Autodesk Inventor part; units mm, degrees
ref_plane "YZ Plane" through (0, 0, 0) normal (1, 0, 0) x (0, 1, 0)
ref_plane "XZ Plane" through (0, 0, 0) normal (0, 1, 0) x (-1, 0, 0)
ref_plane "XY Plane" through (0, 0, 0) normal (0, 0, 1) x (1, 0, 0)
sketch "Sketch1" plane through (0, 0, 0) normal (0, 1, 0) x (-1, 0, 0)
  line L0 (0, 0) -> (-41, 0)
  line L1 (-41, 0) -> (-41, -47)
  line L2 (-41, -47) -> (0, -47)
  line L3 (0, -47) -> (0, 0)
  dimension "d0" = 41
  dimension "d1" = 47
extrude "Extrusion1" add sketch "Sketch1" along normal blind 4
sketch "Sketch2" plane through (0, 4, 0) normal (0, 1, 0) x (1, 0, 0)
  line L0 (41, 47) -> (0, 47) construction
  line L1 (0, 47) -> (0, 0) construction
  line L2 (0, 0) -> (41, 0) construction
  line L3 (41, 0) -> (41, 47) construction
  line L4 (4, 4) -> (4, 43) construction
  line L5 (4, 43) -> (37, 43) construction
  line L6 (37, 43) -> (37, 4) construction
  line L7 (37, 4) -> (4, 4) construction
  line L8 (0, 35.5) -> (4, 35.5)
  line L9 (4, 35.5) -> (4, 27.5)
  line L10 (4, 27.5) -> (0, 27.5)
  line L11 (0, 35.5) -> (0, 27.5)
  line L12 (0, 23.5) -> (41, 23.5) construction
  line L13 (20.5, 0) -> (20.5, 47) construction
  line L14 (41, 47) -> (0, 47) construction
  line L15 (8.5, 47) -> (8.5, 43)
  line L16 (8.5, 43) -> (16.5, 43)
  line L17 (16.5, 43) -> (16.5, 47)
  line L18 (16.5, 47) -> (8.5, 47)
  line L19 (41, 35.5) -> (37, 35.5)
  line L20 (37, 35.5) -> (37, 27.5)
  line L21 (37, 27.5) -> (41, 27.5)
  line L22 (41, 35.5) -> (41, 27.5)
  line L23 (32.5, 47) -> (32.5, 43)
  line L24 (32.5, 43) -> (24.5, 43)
  line L25 (24.5, 43) -> (24.5, 47)
  line L26 (24.5, 47) -> (32.5, 47)
  line L27 (41, 0) -> (0, 0)
  line L28 (4, 4) -> (37, 4)
  line L29 (0, 11.5) -> (4, 11.5)
  line L30 (4, 11.5) -> (4, 19.5)
  line L31 (4, 19.5) -> (0, 19.5)
  line L32 (0, 11.5) -> (0, 19.5)
  line L33 (41, 0) -> (0, 0)
  line L34 (8.5, 0) -> (8.5, 4)
  line L35 (8.5, 4) -> (16.5, 4)
  line L36 (16.5, 4) -> (16.5, 0)
  line L37 (16.5, 0) -> (8.5, 0)
  line L38 (24.5, 4) -> (24.5, 0)
  line L39 (32.5, 0) -> (32.5, 4)
  line L40 (37, 11.5) -> (37, 19.5)
  line L41 (41, 11.5) -> (37, 11.5)
  line L42 (41, 11.5) -> (41, 19.5)
  line L43 (37, 19.5) -> (41, 19.5)
  line L44 (24.5, 0) -> (32.5, 0)
  line L45 (32.5, 4) -> (24.5, 4)
  dimension "d8" = 4
  dimension "d9" = 8
  dimension "d10" = 4
  dimension "d11" = 8
  dimension "d12" = 4
extrude "Extrusion2" cut sketch "Sketch2" against normal up to surface (4 mm away) contours L8 L9 L10 L11 | L18 L17 L16 L15 | L22 L21 L20 L19 | L23 L24 L25 L26 | L27 L38 L28 L39 | L27 L34 L28 L36 | L32 L31 L30 L29 | L40 L43 L42 L41
properties part number "right" material "PBT Plastic Black"
Build history of the part. All positions in model axes, mm. A direction names the side the tool comes from. Coordinates: 2 decimals unless noted, no trailing zeros. Write each loop counter-clockwise with the first axis right and the second up, starting at its lowest first coordinate (ties: lowest second). Pieces come first, ordered by that corner, then holes.
1. Drill centre lines: probe 1 along X at (y, z) = (3.3, -44); probe 2 along Z at (x, y) = (28.5, 3.55); probe 3 along X at (y, z) = (2.7, -30.5). Where is each one in solid material? Low to high.
Answer block:
probe 1: x = 0 to 8.5, 16.5 to 24.5, 32.5 to 41
probe 2: z = -43 to -4
probe 3: x = 4 to 37
2. Band-saw the part on B-B, the plane x = 11. Give the cut face in (y, z), and give its area (3 significant figures).
Answer block:
outline: (0, -43) - (4, -43) - (4, -4) - (0, -4) - close
area: 156 mm2
3. Band-saw the part on C-C, the plane z = -31.5. Give the cut face in (x, y).
Answer block:
outline: (4, 0) - (37, 0) - (37, 4) - (4, 4) - close
4. Drop a flat-ended pin along its axis: pin 1 (2 mm diameter, centred on x = 26.5, y = 3, fed in from -Z). Give the stop position or say it passes through.
Answer block:
pin 1: stops at z = -43
5. 3-axis set-ups, long thin cutter, end or side, ignore diameter. For faces 1 (the flat face through (37, 2, 0)), 2 (the flat face through (28, 2, -4)), 3 (the flat face through (37, 2, -15)), 4 (the flat face through (29, 2, -43)): which of +Z, -Z, +X, -X, +Y, -Y reach the whole face in a straight line?
Answer block:
face 1: +Z, +X, -X, +Y, -Y
face 2: +Z, +Y, -Y
face 3: +X, +Y, -Y
face 4: -Z, +Y, -Y
6. Band-saw the part on A-A, the plane z = -3. Give the cut face in (x, y).
Answer block:
outline: (0, 0) - (8.5, 0) - (8.5, 4) - (0, 4) - close; (16.5, 0) - (24.5, 0) - (24.5, 4) - (16.5, 4) - close; (32.5, 0) - (41, 0) - (41, 4) - (32.5, 4) - close
7. Pull direction Z, two halves, no side cores. Call faces 5 (the flat face through (12, 2, -4)), 6 (the flat face through (32.5, 2, -45)), 7 (the flat face through (4, 2, -15)), 8 (the flat face through (39, 2, -35.5)): released by +Z, released by -Z, zero draft, split by the parting line, or undercut.
Answer block:
face 5: released by +Z
face 6: zero draft
face 7: undercut
face 8: undercut
